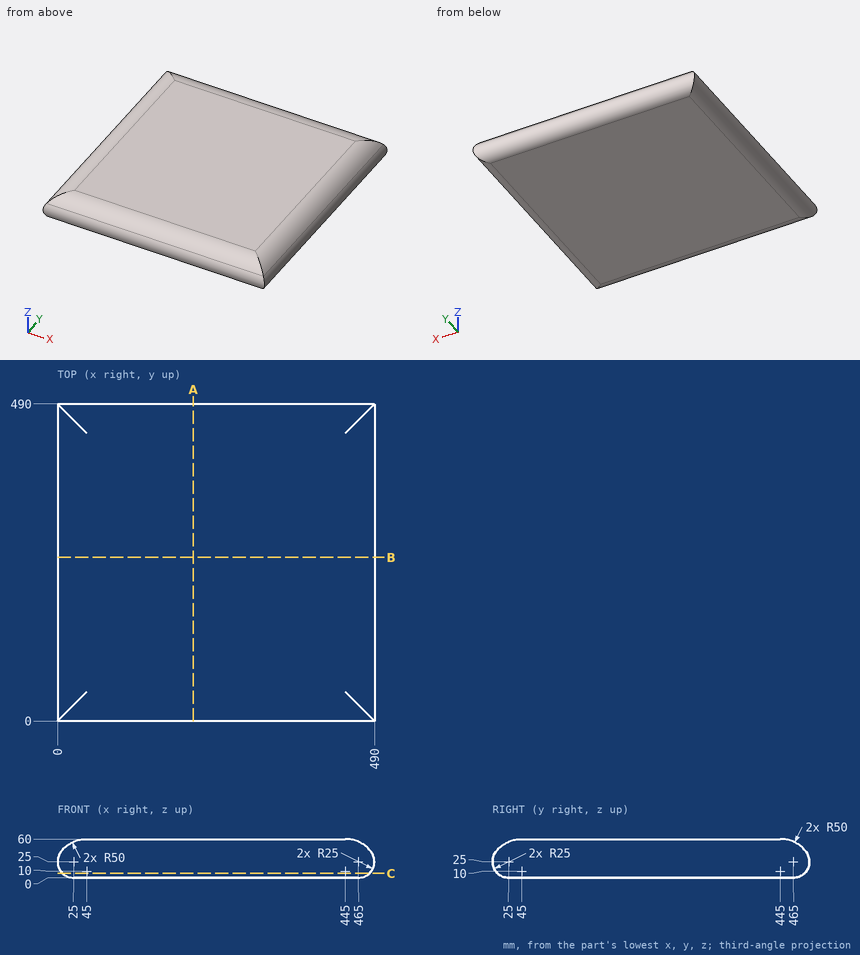
Could you check a few things on this drawing? It's one solid part, dimensions in mm from its lowest x, y, z. Give positions to 0.01 mm unless a question says otherwise; leave off trailing zeros. Loops run counter-clockwise (first coordinate to the right, second up) from the corner with the lowest first, then second, coordinate; pieces in that order, holes last. Notation, with made-up numbers: M 3,-31.75 L 47,-31.75 A27 ccw 47,3.25 Z; hole C -22.5,-25 d7. An arc over 180 degrees is marked long. Answer as a JSON object with one key per item and string values.
Q1. If I drill on probe 1 along Y at (x, z) = (22, 23); probe 2 along Y at (x, z) = (51, 25.5) (3 decimals); probe 3 along X at (y, z) = (272.5, 51), over which ranges is the centre line in solid material (lowest first)? Write a range as [from, to].
Values found:
{"probe 1": "y = [0.08, 489.92]", "probe 2": "y = [0.005, 489.995]", "probe 3": "x = [16.38, 473.62]"}
Q2. Suppose I cut it at C-C, the plane z = 7. List the corners of the cut face in (x, y) for me.
Values found:
{"outline": "M 7.65,7.65 L 482.35,7.65 L 482.35,482.35 L 7.65,482.35 Z"}
Q3. For P1, Ø10, axis at y = 129.5, z = 53, coming from the +X side; P2, Ø12, axis at x = 122.5, z = 43.5, coming from the -Y side; P3, Ø1, axis at y = 438, z = 14.5, coming from the +X side, each with a flat end and sliding along its axis, tell me the tip position at first contact or that it passes through.
Values found:
{"P1": "stops at x = 477.5", "P2": "stops at y = 3.35", "P3": "stops at x = 487.91"}
Q4. Suppose I cut it at A-A, the plane x = 210. List the corners of the cut face in (y, z) for me, plus the area to 3 significant figures.
Values found:
{"outline": "M 5,40 A25 ccw 25,0 L 465,0 A25 ccw 485,40 A50 ccw 445,60 L 45,60 A50 ccw Z", "area": "28,400 mm²"}
